from build123d import *

# Parameters (mm, degrees)
F0_W        = 0.6898511201
F0_H        = 1.2626703829
F0_H_2      = 3.2899174839
F2_DEPTH    = 1.2573
F3_DEPTH    = 2.54
F4_T1_DEPTH = 36.3235808909
F4_T3_DEPTH = 2.5253407657
F4_T5_DEPTH = 2.5253407657


# Not quite as in the source:
# - a fillet or chamfer that OpenCascade refuses, or shapes differently, is made with other operations: its cross-section is extruded or revolved along the edge and cut away or added
# - a feature names something its author has since deleted; it is built from what else it names


with BuildPart() as f1:
    # F0 (on Top) → F1 (revolve)
    with BuildSketch(Plane.XY):
        with BuildLine():
            Line((-19.7332594544, -5.8078670874), (-19.7332594544, -4.5451967046))
            Line((-19.7332594544, -4.5451967046), (-20.5092396879, -4.5451967046))
            ThreePointArc((-20.5092396879, -4.5451967046), (-20.2997388093, -5.2862233267), (-19.7332594544, -5.8078670874))
        make_face()
        with Locations((-19.3883338943, -5.176531896)):
            Rectangle(F0_W, F0_H)
    revolve(axis=Axis((-19.3883338943, -4.5451967046, 0), (1, 0, 0)))



with BuildPart() as f1b:
    # F0 (on Top) → F1, piece 2 (revolve)
    with BuildSketch(Plane.XY):
        with BuildLine():
            Line((20.5092396879, -4.5451967046), (19.7332594544, -4.5451967046))
            Line((19.7332594544, -4.5451967046), (19.7332594544, -5.8078670874))
            ThreePointArc((19.7332594544, -5.8078670874), (20.2997388093, -5.2862233267), (20.5092396879, -4.5451967046))
        make_face()
        with Locations((19.3883338943, -5.176531896)):
            Rectangle(F0_W, F0_H)
    revolve(axis=Axis((-19.3883338943, -4.5451967046, 0), (1, 0, 0)))


with BuildPart() as f1_1:
    add(f1.part)

    add(f1b.part)  # F2 merges F1b
    # F0 (on Top) → F2 (join, symmetric)
    with BuildSketch(Plane.XY):
        Polygon((-20.009059459, 0.0073911622), (-19.7332594544, 0.0073911622), (-19.0434083343, 0.0073911622), (-18.1617904454, 0.0073911622), (-18.1617904454, -5.8078670874), (0, -5.8078670874), (18.1617904454, -5.8078670874), (18.1617904454, 0.0073911622), (19.0434083343, 0.0073911622), (19.7332594544, 0.0073911622), (20.009059459, 0.0073911622), (20.009059459, -3.01362928), (22.5344002247, -3.01362928), (22.5344002247, 39.2609333619), (0, 39.2609333619), (-22.5344002247, 39.2609333619), (-22.5344002247, -3.01362928), (-20.009059459, -3.01362928), align=None)
        with Locations((-19.3883338943, -1.6375675797)):
            Rectangle(F0_W, F0_H_2)
        with Locations((19.3883338943, -1.6375675797)):
            Rectangle(F0_W, F0_H_2)
        with Locations((-19.3883338943, -3.9138615131)):
            Rectangle(F0_W, F0_H)
        with Locations((19.3883338943, -3.9138615131)):
            Rectangle(F0_W, F0_H)
    extrude(amount=F2_DEPTH, both=True)

    # F3 (cut): a face of the model
    f3_faces = [f1_1.faces().sort_by_distance(p)[0] for p in [
        (0, -5.8078670874, 0),
    ]]
    extrude(f3_faces, amount=-F3_DEPTH, mode=Mode.SUBTRACT)

    # F4: fillet of radius 1.27 on 6 edges, made by hand

    # F4_s2 → F4_t1 (cut)
    with BuildSketch(Plane.YZ.offset(-18.1617904454)):
        with BuildLine():
            ThreePointArc((-1.9978670874, 1.2573), (-2.8958926995, 0.8853256121), (-3.2678670874, -0.0127))
            Line((-3.2678670874, -0.0127), (-3.2932670874, -0.0127))
            Line((-3.2932670874, -0.0127), (-3.2932670874, 1.2827))
            Line((-3.2932670874, 1.2827), (-1.9978670874, 1.2827))
            Line((-1.9978670874, 1.2827), (-1.9978670874, 1.2573))
        make_face()
        with BuildLine():
            ThreePointArc((-1.9978670874, -1.2573), (-2.8958926995, -0.8853256121), (-3.2678670874, 0.0127))
            Line((-3.2678670874, 0.0127), (-3.2932670874, 0.0127))
            Line((-3.2932670874, 0.0127), (-3.2932670874, -1.2827))
            Line((-3.2932670874, -1.2827), (-1.9978670874, -1.2827))
            Line((-1.9978670874, -1.2827), (-1.9978670874, -1.2573))
        make_face()
    extrude(amount=F4_T1_DEPTH, mode=Mode.SUBTRACT)

    # F4_s4 → F4_t3 (cut)
    with BuildSketch(Plane.YZ.offset(-22.5344002247)):
        with BuildLine():
            ThreePointArc((-1.74362928, 1.2573), (-2.6416548921, 0.8853256121), (-3.01362928, -0.0127))
            Line((-3.01362928, -0.0127), (-3.03902928, -0.0127))
            Line((-3.03902928, -0.0127), (-3.03902928, 1.2827))
            Line((-3.03902928, 1.2827), (-1.74362928, 1.2827))
            Line((-1.74362928, 1.2827), (-1.74362928, 1.2573))
        make_face()
        with BuildLine():
            ThreePointArc((-1.74362928, -1.2573), (-2.6416548921, -0.8853256121), (-3.01362928, 0.0127))
            Line((-3.01362928, 0.0127), (-3.03902928, 0.0127))
            Line((-3.03902928, 0.0127), (-3.03902928, -1.2827))
            Line((-3.03902928, -1.2827), (-1.74362928, -1.2827))
            Line((-1.74362928, -1.2827), (-1.74362928, -1.2573))
        make_face()
    extrude(amount=F4_T3_DEPTH, mode=Mode.SUBTRACT)

    # F4_s6 → F4_t5 (cut)
    with BuildSketch(Plane.YZ.offset(20.009059459)):
        with BuildLine():
            ThreePointArc((-1.74362928, 1.2573), (-2.6416548921, 0.8853256121), (-3.01362928, -0.0127))
            Line((-3.01362928, -0.0127), (-3.03902928, -0.0127))
            Line((-3.03902928, -0.0127), (-3.03902928, 1.2827))
            Line((-3.03902928, 1.2827), (-1.74362928, 1.2827))
            Line((-1.74362928, 1.2827), (-1.74362928, 1.2573))
        make_face()
        with BuildLine():
            ThreePointArc((-1.74362928, -1.2573), (-2.6416548921, -0.8853256121), (-3.01362928, 0.0127))
            Line((-3.01362928, 0.0127), (-3.03902928, 0.0127))
            Line((-3.03902928, 0.0127), (-3.03902928, -1.2827))
            Line((-3.03902928, -1.2827), (-1.74362928, -1.2827))
            Line((-1.74362928, -1.2827), (-1.74362928, -1.2573))
        make_face()
    extrude(amount=F4_T5_DEPTH, mode=Mode.SUBTRACT)


solid = f1_1.part
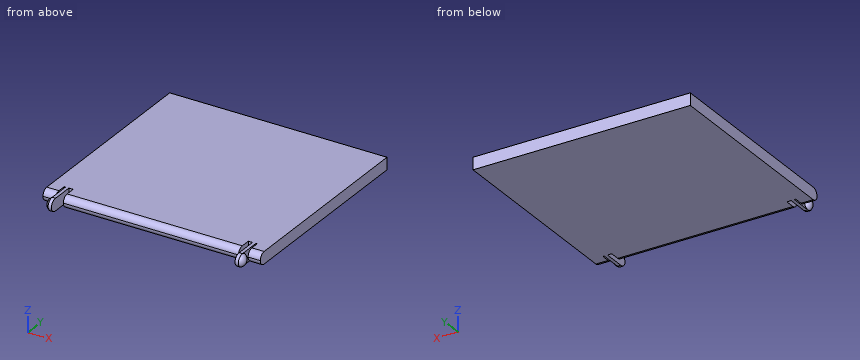
Could you check a few things on this model? Use its own coordinates, in mm. Give positions to 0.01 mm unless a question says otherwise; leave off trailing zeros. Order: outer loops, then holes, each group sorted by start corner. A loop starts at its lowest first (then second) coordinate and runs counter-clockwise, first axis right, second up. Notation, with made-up numbers: (-29, 49.25) -> (25, 49.25) arc R23 ccw to (25, 79.25) -> close; hole circle Ø11 at (42.25, 68.5). An arc over 180 degrees is marked (long way). Answer in a Markdown table with one row per item. Add a question column.
Item 1: Imagine slicing it at A-A (x = -16.5). List the corners of the cut face in (y, z) for me.
Item 2: Imagine slicing it at B-B (z = -0.85). List the corners of the cut face in (x, y) for me, and give its area (3 significant figures).
Item 3: I'm going to push flat-ended pins straight in: P1, Ø22, axis at x = -11, y = 23.5, coming from the +Z side; P2, Ø12, axis at x = -1, y = 4, coming from the -Z side. Where does each tip first touch, or does it pass through?
Item 4: Please list where these lines run through material, in increasing order: probe 1 along X at (y, z) = (-3, 0.95); probe 2 along Y at (x, z) = (-10, 0.1); probe 3 along Z at (x, y) = (-12.5, 37).
Result:
| question | item | result |
|---|---|---|
| 1 | outline | (-3.27, 0) arc R1.27 ccw to (-2, -1.26) -> (39.26, -1.26) -> (39.26, 1.26) -> (-2, 1.26) arc R1.27 ccw to start |
| 2 | outline | (-22.53, -2.68) -> (-20.01, -2.68) -> (-20.01, 0.01) -> (-19.73, 0.01) -> (-19.73, -3.61) arc R1.13 ccw to (-19.73, -5.48) -> (-19.04, -5.48) -> (-19.04, 0.01) -> (-18.16, 0.01) -> (-18.16, -2.93) -> (18.16, -2.93) -> (18.16, 0.01) -> (19.04, 0.01) -> (19.04, -5.48) -> (19.73, -5.48) arc R1.13 ccw to (19.73, -3.61) -> (19.73, 0.01) -> (20.01, 0.01) -> (20.01, -2.68) -> (22.53, -2.68) -> (22.53, 39.26) -> (-22.53, 39.26) -> close |
| 2 | area | 1,900 mm2 |
| 3 | P1 | z = 1.26 |
| 3 | P2 | z = -1.26 |
| 4 | probe 1 | -19.73 to -19.04, 19.04 to 19.73 |
| 4 | probe 2 | -3.26 to 39.26 |
| 4 | probe 3 | -1.26 to 1.26 |
